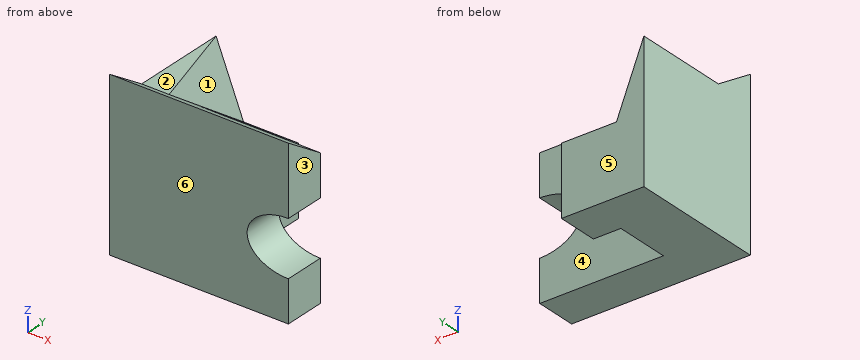
```python
from build123d import *

# Parameters (mm, degrees)
BOSS_EXTRUDE1_DEPTH = 65
BOSS_EXTRUDE2_DEPTH = 20
BOSS_EXTRUDE3_DEPTH = 30
BOSS_EXTRUDE4_DEPTH = 10
CUT_EXTRUDE1_DEPTH  = 10
CUT_EXTRUDE3_REACH  = 97.131
SKETCH3_RX          = 15
SKETCH3_RY          = 10


with BuildPart() as part:
    # Sketch1 → Boss-Extrude1 (new body)
    with BuildSketch(Plane(origin=(0, 0, 0), x_dir=(0, 0, -1), z_dir=(1, 0, 0))):
        Polygon((-60, 0), (-50, 15), (0, 15), (0, 0), align=None)
    extrude(amount=BOSS_EXTRUDE1_DEPTH)

    # Sketch1_3 → Boss-Extrude2 (add)
    with BuildSketch(Plane(origin=(0, 0, 0), x_dir=(0, 0, -1), z_dir=(1, 0, 0))):
        Polygon((-50, 15), (0, 15), (0, 35), (-35.714285714, 35), align=None)
    extrude(amount=BOSS_EXTRUDE2_DEPTH)

    # Sketch1_4 → Boss-Extrude3 (add)
    with BuildSketch(Plane(origin=(0, 0, 0), x_dir=(0, 0, -1), z_dir=(1, 0, 0))):
        Polygon((-35.714285714, 35), (0, 35), (0, 50), (-25, 50), align=None)
    extrude(amount=BOSS_EXTRUDE3_DEPTH)

    # Sketch1_5 → Boss-Extrude4 (add)
    with BuildSketch(Plane(origin=(0, 0, 0), x_dir=(0, 0, -1), z_dir=(1, 0, 0))):
        Polygon((-50, 50), (-50, 15), (-35.714285714, 35), (-25, 50), align=None)
    extrude(amount=BOSS_EXTRUDE4_DEPTH)

    # Sketch2 → Cut-Extrude1 (cut, along a direction that is not the sketch's normal)
    with BuildSketch(Plane(origin=(27.613412229, 7.889546351, 11.045364892), x_dir=(-0.3451624427428596, -0.09861784078367415, 0.9333474217026305), z_dir=(-0.8974358974358975, -0.2564102564102566, -0.358974358974359))):
        Polygon((41.736479046, 48.076197382), (14.951169076, 45.328986103), (41.736479046, 11.675647936), align=None)
    extrude(amount=-CUT_EXTRUDE1_DEPTH, dir=(-1, 0, 0), mode=Mode.SUBTRACT)

    # Sketch3 → Cut-Extrude3 (cut, up to next)
    with BuildSketch(Plane(origin=(0, 15, 0), x_dir=(1, 0, 0), z_dir=(0, 1, 0)), mode=Mode.PRIVATE) as cut_extrude3_sk1:
        with Locations((65, -25)):
            Ellipse(SKETCH3_RX, SKETCH3_RY)
    cut_extrude3_tool1 = extrude(cut_extrude3_sk1.sketch, amount=-CUT_EXTRUDE3_REACH, mode=Mode.PRIVATE) & part.part
    add(cut_extrude3_tool1.solids().sort_by_distance((65, 15, 25))[0], mode=Mode.SUBTRACT)


solid = part.part
```
CAD build for the part. Positions are in the model's coordinates, mm. Face numbers are marked on the shaded views. A direction names the side the tool comes from. Give positions to 0.01 mm unless a question says otherwise; leave off trailing zeros. Loops run counter-clockwise (first coordinate to the right, second up) from the corner with the lowest first, then second, coordinate; pieces in that order, holes last. Notation, with made-up numbers: (46, 26.25) -> (66, 26.25) arc R14 ccw to (66, 33.25) -> close; hole circle Ø3 at (71.25, -11.5). An arc over 180 degrees is marked (long way). Use a Markdown table: item, result.
1. Slice it at C-C (y = 42). List the corners of the cut face in (x, z), plus the area to 3 significant figures.
Check result:
| item | result |
|---|---|
| outline | (0, 0) -> (30, 0) -> (30, 30.71) -> (10, 30.71) -> (2.29, 50) -> (0, 50) -> close |
| area | 1,040 mm^2 |
2. Slice it at A-A (x = 5). List the corners of the cut face in (y, z).
Check result:
| item | result |
|---|---|
| outline | (0, 0) -> (50, 0) -> (50, 37.5) -> (32.5, 50) -> (15, 50) -> (0, 60) -> close |
3. Which spindle directions (+Z, -Z, +X, -X, +Y, -Y) get a long thin tool onto all of the face, cutting with end or side? Do the marked faces 1 and 2. Say none if no direction does.
Check result:
| item | result |
|---|---|
| face 1 | +Z, +X, +Y |
| face 2 | +Z, +X, -X, +Y |
4. Wall check: L1, parallel to X at y = 30.5, z = 13; L2, parallel to Y at x = 35, z = 20; L3, parallel to X at y = 35.5, z = 28. Give the ranges that are in metal, low to high. Write a range as [from, to].
Check result:
| item | result |
|---|---|
| L1 | x = [0, 20] |
| L2 | y = [0, 15] |
| L3 | x = [0, 30] |
5. Slice it at B-B (z = 39.5). List the corners of the cut face in (x, y).
Check result:
| item | result |
|---|---|
| outline | (0, 0) -> (65, 0) -> (65, 15) -> (20, 15) -> (20, 29.7) -> (10, 29.7) -> (4.2, 50) -> (0, 50) -> close |
6. Mould opens along Y. For the marked faces 3, 4, 5 and 6 say: pulls with the +Y half, pulls with the -Y half, needs draft (parallel to the pull), parting line crosses it, or undercut.
Check result:
| item | result |
|---|---|
| face 3 | needs draft |
| face 4 | undercut |
| face 5 | pulls with the +Y half |
| face 6 | pulls with the -Y half |
7. Flat gauge pins, fed straight in: pin 1 (4 mm diameter, centred on x = 42, z = 42, fed in from +Y); pin 2 (5 mm diameter, centred on x = 33.5, y = 7.5, fed in from +Z); pin 3 (8 mm diameter, centred on x = 3.5, y = 40, fed in from +Z). Where does each tip first touch, or does it go through?
Check result:
| item | result |
|---|---|
| pin 1 | stops at y = 15 |
| pin 2 | stops at z = 56.67 |
| pin 3 | stops at z = 50 |
8. Slice it at D-D (z = 56.5). List the corners of the cut face in (x, y), plus the area to 3 significant figures.
Check result:
| item | result |
|---|---|
| outline | (0, 0) -> (65, 0) -> (65, 5.25) -> (0, 5.25) -> close |
| area | 341 mm^2 |
